Study the drawing (mm; zero at the part's minimum x, y, z) and answer. A direction names the side the tool comes from. Give positions to 0.01 mm unless a question says otherwise; leave off trailing zeros. Write each loop counter-clockwise with the first axis right and the second up, starting at its lowest first coordinate (ties: lowest second). Pieces come first, ordered by that corner, then holes. Notation, with made-up numbers: (57.25, -34.5) - (101.25, -34.5) arc R27 ccw to (101.25, -14.5) - close; hole circle Ø9 at (68.25, 57.25). An arc over 180 degrees is marked (long way). Write each question's results on one line, items separated by ' | '. Start each with the question number.
Q1. Find the intervals of material crossed by probe 1 along X at (y, z) = (6.75, 6.35); probe 2 along Z at (x, y) = (3.5, 8.75); probe 3 along X at (y, z) = (7.5, 6), in increasing order.
Q2. A flat-ended cylindrical pin translates along its axis: pin 1 Ø4 at (x, y) = (18, 4.5) entering from -Z. Find the tip coordinate at first contact, or state that the pin passes through.
Q3. For the marked faces 4, 5 and 6, determine the directions among +Z, -Z, +X, -X, +Y, -Y from which every point of the face is accessible in a straight line to the end or side of a thin tool.
Q4. Section B-B (x = 26) is taken. Determine the outline of the cut face in (y, z), plus the area to 3 significant figures.
Q5. Section C-C (y = 2.5) is taken. Determine the outline of the cut face in (x, z), plus the area to 3 significant figures.
Q6. Section A-A (z = 6.35) is taken. Determine the outline of the cut face in (x, y), plus the area to 3 significant figures.
Q7. For a pull along X with two mould halves and no side action, classify the marked faces 1, 2 and 3 as pulls with the +X half, pulls with the -X half, needs draft (parallel to the pull), parting line crosses it, or undercut.
Q8. Section D-D (x = 15) is taken. Determine the outline of the cut face in (y, z).
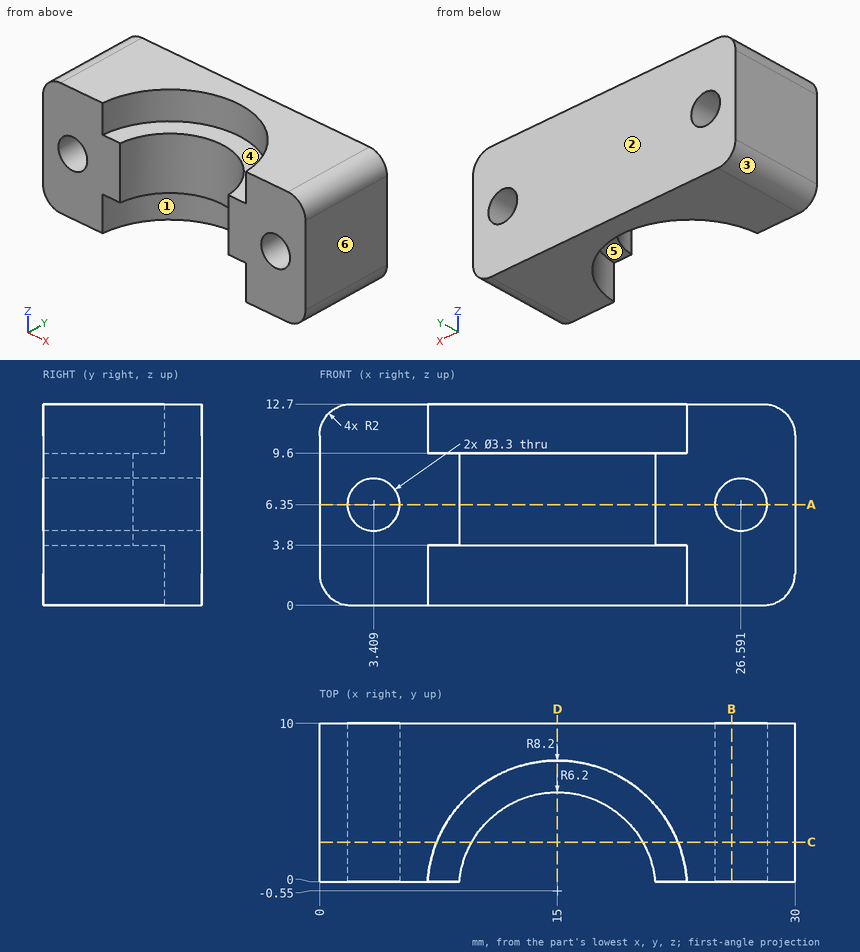
Answers below:
1) probe 1: x = 0 to 1.76, 5.06 to 24.94, 28.24 to 30 | probe 2: z = 0 to 4.7, 8 to 12.7 | probe 3: x = 0 to 1.8, 5.02 to 24.98, 28.2 to 30
2) pin 1: stops at z = 3.8
3) face 4: +Z, -Y | face 5: -Z, -Y | face 6: +Z, -Z, +X, +Y, -Y
4) outline: (0, 0) - (10, 0) - (10, 4.81) - (0, 4.81) - close; (0, 7.89) - (10, 7.89) - (10, 12.7) - (0, 12.7) - close | area: 96.2 mm2
5) outline: (0, 2) arc R2 ccw to (2, 0) - (7.39, 0) - (7.39, 3.8) - (9.6, 3.8) - (9.6, 9.6) - (7.39, 9.6) - (7.39, 12.7) - (2, 12.7) arc R2 ccw to (0, 10.7) - close; (20.4, 3.8) - (22.61, 3.8) - (22.61, 0) - (28, 0) arc R2 ccw to (30, 2) - (30, 10.7) arc R2 ccw to (28, 12.7) - (22.61, 12.7) - (22.61, 9.6) - (20.4, 9.6) - close; hole circle Ø3.3 at (3.41, 6.35); hole circle Ø3.3 at (26.59, 6.35) | area: 193 mm2
6) outline: (0, 0) - (1.76, 0) - (1.76, 10) - (0, 10) - close; (5.06, 0) - (8.82, 0) arc R6.2 cw to (21.18, 0) - (24.94, 0) - (24.94, 10) - (5.06, 10) - close; (28.24, 0) - (30, 0) - (30, 10) - (28.24, 10) - close | area: 180 mm2
7) face 1: undercut | face 2: needs draft | face 3: pulls with the -X half
8) outline: (5.65, 3.8) - (7.65, 3.8) - (7.65, 0) - (10, 0) - (10, 12.7) - (7.65, 12.7) - (7.65, 9.6) - (5.65, 9.6) - close
